The listing builds one solid part. Answer for the finished solid, in the listing's coordinates (mm). A direction names the side the tool comes from. Round coordinates to 2 decimals unless told otherwise and drop trailing zeros. Loops run counter-clockwise (first coordinate to the right, second up) from the corner with the lowest first, then second, coordinate; pieces in that order, holes last. Notation, with made-up numbers: (34.25, -21.75) - (60.25, -21.75) arc R20 cw to (60.25, 14.25) - close; hole circle Ø4 at (-17, 0.25). An arc over 180 degrees is marked (long way). One line per question, with ' | ' between items. Start each with the question number.
from build123d import *

# Parameters (mm, degrees)
SKETCH1_R      = 6.05
SKETCH1_R_2    = 5.55
EXTRUDE1_DEPTH = 49
SKETCH2_R      = 10.5
SKETCH2_R_2    = 5.5
EXTRUDE3_DEPTH = 2
EXTRUDE4_START = 2
SKETCH3_R      = 10.5
SKETCH3_R_2    = 5.5
EXTRUDE4_DEPTH = 2


with BuildPart() as part:
    # Sketch1 → Extrude1 (new body)
    with BuildSketch(Plane.XY):
        Circle(SKETCH1_R)
        Circle(SKETCH1_R_2, mode=Mode.SUBTRACT)
    extrude(amount=EXTRUDE1_DEPTH)

    # Sketch2 → Extrude3 (add)
    with BuildSketch(Plane.XY.offset(49)):
        Circle(SKETCH2_R)
        Circle(SKETCH2_R_2, mode=Mode.SUBTRACT)
    extrude(amount=EXTRUDE3_DEPTH)

    # Sketch3 → Extrude4 (add)
    with BuildSketch(Plane(origin=(0, 0, 0), x_dir=(-1, 0, 0), z_dir=(0, 0, -1)).offset(EXTRUDE4_START)):
        with Locations(Location((0, 0, 0), (0, 0, 180))):
            Circle(SKETCH3_R)
        with Locations(Location((0, 0, 0), (0, 0, 180))):
            Circle(SKETCH3_R_2, mode=Mode.SUBTRACT)
    extrude(amount=-EXTRUDE4_DEPTH)


solid = part.part
(1) Find section A-A on y = 0. Write down the section's boundary in (x, z), plus the area to 3 significant figures.
(2) Find section C-C on z = 46. Write down the section's boundary in (x, y), plus the area to 3 significant figures.
(3) Each of these flat-tipped pins is pushed along its axis until it touches: P1, Ø5, axis at y = 0.5, z = 31, coming from the +X side; P2, Ø3, axis at x = -8, z = 28, coming from the +Y side; P3, Ø2, axis at y = 4, z = 41.5, coming from the +X side; P4, Ø1, axis at x = -6, z = 28, coming from the -Y side. Where does it stop, or does it pass through?
(4) Consider L1, parallel to Z at x = 3.25, y = -9.25; L2, parallel to Y at x = 0, z = 24.5; L3, parallel to Y at x = 0, z = 50.4. Determine where each line is inside the solid, lowest interval first.
(5) Determine the mould class of faces 1 (the cylindrical face through (2.98, 4.68, 24.16)), 2 (the flat face through (5, -5, 51)), 3 (the cylindrical face through (10, -3.2, -1)), 4 (the cylindrical face through (-1.19, -5.37, 49.99)) for opening direction X: pulls with the +X half, pulls with the -X half, needs draft (parallel to the pull), parting line crosses it, or undercut.
(6) A tool of negligible diameter and unlimited length cuts with its end or side. For faces 5 (the flat face through (5, 5, -2)), 6 (the cylindrical face through (5.589, -2.317, 24.157)), from which of +Z, -Z, +X, -X, +Y, -Y can it reach the whole face along a straight path? Write none if from no direction.
(7) Find section D-D on x = -7.25. Write down the section's boundary in (y, z).
Answer below:
1) outline: (-10.5, -2) - (-5.5, -2) - (-5.5, 0) - (-5.55, 0) - (-5.55, 49) - (-5.5, 49) - (-5.5, 51) - (-10.5, 51) - (-10.5, 49) - (-6.05, 49) - (-6.05, 0) - (-10.5, 0) - close; (5.5, -2) - (10.5, -2) - (10.5, 0) - (6.05, 0) - (6.05, 49) - (10.5, 49) - (10.5, 51) - (5.5, 51) - (5.5, 49) - (5.55, 49) - (5.55, 0) - (5.5, 0) - close | area: 89.0 mm2
2) outline: circle Ø12.1 at (0, 0); hole circle Ø11.1 at (0, 0) | area: 18.2 mm2
3) P1: x = 6.05 | P2: through | P3: x = 5.25 | P4: y = -2.52
4) L1: -2 to 0, 49 to 51 | L2: -6.05 to -5.55, 5.55 to 6.05 | L3: -10.5 to -5.5, 5.5 to 10.5
5) face 1: undercut | face 2: needs draft | face 3: parting line crosses it | face 4: undercut
6) face 5: -Z, +X, -X, +Y, -Y | face 6: none
7) outline: (-7.6, -2) - (7.6, -2) - (7.6, 0) - (-7.6, 0) - close; (-7.6, 49) - (7.6, 49) - (7.6, 51) - (-7.6, 51) - close
